Input: part model. Units: mm. Frame: model coordinates. A direction names the side the tool comes from. Round coordinates to 2 decimals unless told otherwise and drop trailing zeros. Loops run counter-clockwise (first coordinate to the right, second up) from the corner with the lowest first, then second, coordinate; pieces in that order, holes last. Notation, with made-up numbers: (80.25, -27.5) - (99.25, -27.5) arc R3 ccw to (99.25, -23.5) - close; hole circle Ø11 at (64, -29.75). An arc over 180 degrees is marked (long way). Write each question's results on one line, items separated by ' | '.
Autodesk Inventor part; units mm, degrees
ref_plane "YZ Plane" through (0, 0, 0) normal (1, 0, 0) x (0, 1, 0)
ref_plane "XZ Plane" through (0, 0, 0) normal (0, 1, 0) x (-1, 0, 0)
ref_plane "XY Plane" through (0, 0, 0) normal (0, 0, 1) x (1, 0, 0)
sketch "Sketch1" plane through (0, 0, 0) normal (0, 1, 0) x (-1, 0, 0)
  line L0 (0, 0) -> (150, 0)
  line L1 (150, 0) -> (150, -10)
  line L2 (150, -10) -> (0, -10)
  line L3 (0, -10) -> (0, 0)
  line L4 (144.6787, -5) -> (169.2898, -5)
  line L5 (150, 0) -> (150, 8)
  line L6 (150, 8) -> (169.2898, -5)
  line L7 (150, -10) -> (150, -18)
  line L8 (150, -18) -> (169.2898, -5)
  line L9 (0, -7.6) -> (3.1367, -7.6)
  line L10 (3.1367, -7.6) -> (3.1367, -9.1799)
  line L11 (3.1367, -9.1799) -> (8.1367, -9.1799)
  line L12 (8.1367, -9.1799) -> (8.1367, -5)
  line L13 (0, -2.4) -> (3.1367, -2.4)
  line L14 (3.1367, -2.4) -> (3.1367, -0.8201)
  line L15 (3.1367, -0.8201) -> (8.1367, -0.8201)
  line L16 (8.1367, -0.8201) -> (8.1367, -5)
  line L17 (12.6825, 0) -> (12.6825, 6.9857)
  line L18 (12.6825, 6.9857) -> (0, 6.9857)
  line L19 (0, 6.9857) -> (0, -2.4)
  line L20 (12.6825, -10) -> (12.6825, -16.9857)
  line L21 (12.6825, -16.9857) -> (0, -16.9857)
  line L22 (0, -16.9857) -> (0, -7.6)
  point P0 (0, -2.4)
  point P1 (1.5684, -7.6)
  point P2 (1.5684, -2.4)
  point P3 (3.1367, -1.61)
  dimension "d0" = 10
  dimension "d1" = 150
  dimension "d2" = 8
  dimension "d3" = 5
  dimension "d6" = 5.2
  dimension "d7" = 5
extrude "Extrusion1" add sketch "Sketch1" along normal blind 10 contours L19 L18 L17 L0 | L0 L1 L2 L3 L9 L10 L11 L12 L16 L15 L14 L13 | L5 L6 L4 L1 | L4 L8 L7 L1 | L2 L20 L21 L22
properties part number "Vector" material "Wood (Birch)"
1. Set-up query: faces 1 (the flat face through (-6, 5, -9.18)), 2 (the flat face through (-2, 5, -2.4)), 3 (the flat face through (-6, 5, -16.986)), 4 (the flat face through (-150, 5, 4)). Return all of +Z, -Z, +X, -X, +Y, -Y with unobstructed straight access to the full face (end or side cutting, diameter ignored); none if empty.
Answer:
face 1: +Y, -Y | face 2: +X, +Y, -Y | face 3: -Z, +X, +Y, -Y | face 4: +Z, +Y, -Y
2. Section query B-B, the plane y = 1.75. Output: boundary loops of the cut face in (x, z).
Answer:
outline: (-169.29, -5) - (-150, -18) - (-150, -10) - (-12.68, -10) - (-12.68, -16.99) - (0, -16.99) - (0, -7.6) - (-3.14, -7.6) - (-3.14, -9.18) - (-8.14, -9.18) - (-8.14, -0.82) - (-3.14, -0.82) - (-3.14, -2.4) - (0, -2.4) - (0, 6.99) - (-12.68, 6.99) - (-12.68, 0) - (-150, 0) - (-150, 8) - close
3. Contact query for flat-ended pins moving along their axis: pin 1 (1.3 mm diameter, centred on y = 5.5, z = -8, fed in from -X); pin 2 (1.5 mm diameter, centred on y = 4, z = 2.5, fed in from -X); pin 3 (5.5 mm diameter, centred on y = 6, z = 2.5, fed in from -X). Output: stop coordinate, or through.
Answer:
pin 1: x = -165.8 | pin 2: x = -159.27 | pin 3: x = -162.24
4. Mould query, pull axis Z, two halves, no side actions, for faces 5 (the flat face through (-82, 5, -10)), 6 (the flat face through (-2, 5, -7.6)), 7 (the flat face through (-150, 5, -14)). Classes: pulls with the +Z half, pulls with the -Z half, needs draft (parallel to the pull), parting line crosses it, or undercut.
Answer:
face 5: pulls with the -Z half | face 6: undercut | face 7: needs draft
5. Section query A-A, the plane z = -14.25. Output: boundary loops of the cut face in (x, y).
Answer:
outline: (-155.56, 0) - (-150, 0) - (-150, 10) - (-155.56, 10) - close; (-12.68, 0) - (0, 0) - (0, 10) - (-12.68, 10) - close
6. Section query C-C, the plane x = -37. Output: boundary loops of the cut face in (y, z), plus the area to 3 significant figures.
Answer:
outline: (0, -10) - (10, -10) - (10, 0) - (0, 0) - close | area: 100 mm^2
7. Line query: line 1 (Z direction, x = -141.5, y = 4.25); line 2 (X direction, y = 9, z = 1.25); line 3 (Z direction, x = -9.5, y = 1.75). Output: solid intervals per line, ascending. Write a range as [from, to].
Answer:
line 1: [-10, 0] | line 2: [-160.02, -150], [-12.68, 0] | line 3: [-16.99, 6.99]
